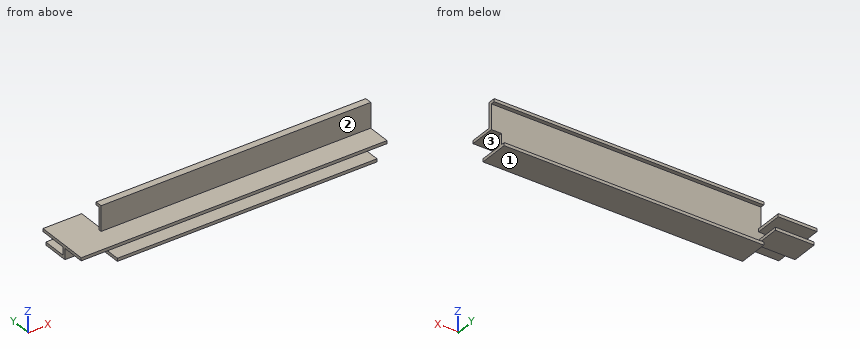
from build123d import *

# Parameters (mm, degrees)
SKETCH1_W                = 1.5
SKETCH1_H                = 2
BOSS_EXTRUDE1_DEPTH      = 259.69214
RIGHT_EAR_DEPTH          = 1.27
RIGHT_EAR_DEPTH_BACK     = 24.45893
SKETCH9_W                = 1.5
SKETCH9_H                = 11.5
LEFT_EAR_DEPTH           = 18.10893
LEFT_EAR_DEPTH_BACK      = 1.27
CUT_EXTRUDE6_DEPTH       = 280.89897194
CUT_EXTRUDE6_DEPTH_BACK  = 280.89897194
SURFACE_EXTRUDE1_1_BACK  = 307.34
SURFACE_EXTRUDE1_1_DEPTH = 308.93893
SURFACE_EXTRUDE1_2_BACK  = 307.34
SURFACE_EXTRUDE1_2_DEPTH = 308.93893
CUT_EXTRUDE7_DEPTH       = 157.732995968


with BuildPart() as part:
    # Sketch1 → Boss-Extrude1 (new body)
    with BuildSketch(Plane(origin=(0, 0, 0), x_dir=(0, 0, -1), z_dir=(1, 0, 0))):
        Polygon((-21, 0), (0, 0), (0, -13), (-1.5, -13), (-1.5, -1.5), (-7, -1.5), (-7, -13), (-8.5, -13), (-8.5, -1.5), (-21, -1.5), align=None)
        with Locations((-20.25, 1)):
            Rectangle(SKETCH1_W, SKETCH1_H)
        with Locations((-0.75, 1)):
            Rectangle(SKETCH1_W, SKETCH1_H)
    extrude(amount=-BOSS_EXTRUDE1_DEPTH)


with BuildPart() as body_2:
    # Mirror3: mirrored copy
    add(part.part.mirror(Plane.ZX.offset(7)))


with BuildPart() as part_1:
    add(part.part)

    add(body_2.part)  # right_ear merges body 2
    # Sketch9 → right_ear (add, two sides: drawn at the far end of the back side and taken through both)
    with BuildSketch(Plane.ZY.offset(-RIGHT_EAR_DEPTH_BACK)):
        with Locations((7.75, -7.25)):
            Rectangle(SKETCH9_W, SKETCH9_H)
        Polygon((1.5, -1.5), (7, -1.5), (8.5, -1.5), (8.5, 15.5), (7, 15.5), (1.5, 15.5), align=None)
        with Locations((7.75, 21.25)):
            Rectangle(SKETCH9_W, SKETCH9_H)
    extrude(amount=RIGHT_EAR_DEPTH + RIGHT_EAR_DEPTH_BACK)

    # Sketch12 → left_ear (add, two sides: drawn at the far end of the back side and taken through both)
    with BuildSketch(Plane.ZY.offset(259.69214).offset(-LEFT_EAR_DEPTH_BACK)):
        Polygon((8.5, -13), (8.5, 27), (7, 27), (7, 15.5), (1.5, 15.5), (1.5, -1.5), (7, -1.5), (7, -13), align=None)
    extrude(amount=LEFT_EAR_DEPTH + LEFT_EAR_DEPTH_BACK)

    # Sketch10<3> → Cut-Extrude6 (cut, two sides: drawn at the far end of the back side and taken through both)
    with BuildSketch(Plane(origin=(0, 0, 0), x_dir=(1, 0, 0), z_dir=(0, 1, 0)).offset(-CUT_EXTRUDE6_DEPTH_BACK)):
        Polygon((-1.27, -1.5), (-129.84607, -1.5), (-129.84607, -7), (-124.84607, -7), (-124.84607, -19.5), (0, -19.5), (0, -8.5), (-1.27, -8.5), align=None)
        Polygon((-129.84607, 5.228694749), (-129.84607, 0), (-129.84607, -1.5), (-1.27, -1.5), (-1.27, -8.5), (0, -8.5), (0, -19.5), (-124.84607, -19.5), (-124.84607, -21), (-124.84607, -30.387985995), (75.346094687, -30.387985995), (75.346094687, 5.228694749), align=None)
    extrude(amount=CUT_EXTRUDE6_DEPTH + CUT_EXTRUDE6_DEPTH_BACK, mode=Mode.SUBTRACT)


with BuildPart() as body_2_2:
    # L-Split2: the piece behind the surface
    add(part_1.part)
    # Surface-Extrude1: a surface, the sketch's curves swept straight by 308.93893 mm
    with BuildLine(Plane(origin=(24.45893, 0, 0), x_dir=(0, 0, -1), z_dir=(1, 0, 0)).offset(-SURFACE_EXTRUDE1_1_BACK), mode=Mode.PRIVATE) as surface_extrude1_1_path:
        Line((-19.5, 14), (-7, 14))
        Line((-7, 14), (-7, 0))
        Line((-7, 0), (-3, 0))
        Line((-3, 0), (-3, 12))
        Line((-3, 12), (0, 12))
    surface_extrude1_1 = Shell.extrude(surface_extrude1_1_path.wire(), (1 * SURFACE_EXTRUDE1_1_DEPTH, 0 * SURFACE_EXTRUDE1_1_DEPTH, 0 * SURFACE_EXTRUDE1_1_DEPTH))
    split(bisect_by=surface_extrude1_1, keep=Keep.BOTTOM)


with BuildPart() as part_2:
    add(part_1.part)

    # L-Split2: split by a surface, the side it looks to stays
    # Surface-Extrude1: a surface, the sketch's curves swept straight by 308.93893 mm
    with BuildLine(Plane(origin=(24.45893, 0, 0), x_dir=(0, 0, -1), z_dir=(1, 0, 0)).offset(-SURFACE_EXTRUDE1_2_BACK), mode=Mode.PRIVATE) as surface_extrude1_2_path:
        Line((-19.5, 14), (-7, 14))
        Line((-7, 14), (-7, 0))
        Line((-7, 0), (-3, 0))
        Line((-3, 0), (-3, 12))
        Line((-3, 12), (0, 12))
    surface_extrude1_2 = Shell.extrude(surface_extrude1_2_path.wire(), (1 * SURFACE_EXTRUDE1_2_DEPTH, 0 * SURFACE_EXTRUDE1_2_DEPTH, 0 * SURFACE_EXTRUDE1_2_DEPTH))
    split(bisect_by=surface_extrude1_2, keep=Keep.TOP)


with BuildPart() as cut_extrude7_tool:
    # Sketch14 → Cut-Extrude7 (new, through all)
    with BuildSketch(Plane.ZY.offset(277.80107)):
        Polygon((-4.726079356, 11.992451092), (3, 12), (3, 0), (7, 0), (7, 14), (19.5, 14), (19.5, 12), (27.004136279, 12), (27.004136279, 32.441536758), (-4.726079356, 32.441536758), align=None)
    extrude(amount=-CUT_EXTRUDE7_DEPTH)


with BuildPart() as part_3:
    add(part_2.part)

    # Cut-Extrude7: cut by cut_extrude7_tool
    add(cut_extrude7_tool.part, mode=Mode.SUBTRACT)


with BuildPart() as body_2_2_1:
    add(body_2_2.part)

    # Cut-Extrude7: cut by cut_extrude7_tool
    add(cut_extrude7_tool.part, mode=Mode.SUBTRACT)


solid = body_2_2_1.part
Design review of the part built by this model. Coordinates are the model's own, in mm. Face numbers are marked on the shaded views. Round coordinates to 2 decimals unless told otherwise and drop trailing zeros. Write each loop counter-clockwise with the first axis right and the second up, starting at its lowest first coordinate (ties: lowest second). Pieces come first, ordered by that corner, then holes. Notation, with made-up numbers: (61, -29) - (89, -29) arc R23 cw to (89, 10) - close; hole circle Ø11 at (-12, 30). An arc over 180 degrees is marked (long way). Use a Markdown table: item, result. Add a question column.
1. We need section D-D (z = 14.5). State the section outline as (x, y) points.
2. We need section A-A (y = -6). State the section outline as (x, z) points.
3. Wall thickness on probe 1 along Z at (x, y) = (-195.5, 0.75); probe 2 along Z at (x, y) = (-254, -2.75); probe 3 along Y at (x, z) = (-223, 17.75): over which ranges is each line inside the solid? List them lowest first.
4. Mouldability with a two-part tool opening along Z and no side actions: class the marked faces 1, 2 and 3 as +Z half, -Z half, draft (parallel to the pull), parting line (faces both ways), or undercut.
5. We need section C-C (y = 6.75). State the section outline as (x, z) points, then the cut area to 3 significant figures.
6. We need section B-B (x = -267). State the section outline as (y, z) points.
7. Clearance check with flat-ended pins moving along their axes: pin 1 (1 mm diameter, centred on x = -219, z = 9.5, fed in from +Y); pin 2 (9 mm diameter, centred on x = -175.5, y = -8, fed in from +Z); pin 3 (4 mm diameter, centred on x = -242.5, z = 11, fed in from -Y); pin 4 (1 mm diameter, centred on x = -176.5, y = 3, fed in from +Z). State where each tip first meets the part, or that it passes through.
Output:
| question | item | result |
|---|---|---|
| 1 | outline | (-259.69, -1.5) - (-124.85, -1.5) - (-124.85, 0) - (-259.69, 0) - close |
| 2 | outline | (-277.8, 7) - (-124.85, 7) - (-124.85, 8.5) - (-277.8, 8.5) - close; (-259.69, 0) - (-129.85, 0) - (-129.85, 1.5) - (-259.69, 1.5) - close |
| 3 | probe 1 | z = 0 to 1.5, 19.5 to 21 |
| 3 | probe 2 | z = 0 to 1.5, 7 to 8.5 |
| 3 | probe 3 | y = -1.5 to 0 |
| 4 | face 1 | -Z half |
| 4 | face 2 | draft |
| 4 | face 3 | undercut |
| 5 | outline | (-277.8, 1.5) - (-258.42, 1.5) - (-258.42, 3) - (-277.8, 3) - close; (-277.8, 7) - (-258.42, 7) - (-258.42, 8.5) - (-277.8, 8.5) - close |
| 5 | area | 58.1 mm2 |
| 6 | outline | (-13, 7) - (-1.5, 7) - (-1.5, 1.5) - (12, 1.5) - (12, 3) - (0, 3) - (0, 7) - (14, 7) - (14, 8.5) - (-13, 8.5) - close |
| 7 | pin 1 | stops at y = 0 |
| 7 | pin 2 | stops at z = 8.5 |
| 7 | pin 3 | stops at y = -1.5 |
| 7 | pin 4 | passes through |
